Autodesk Inventor part; units mm, degrees
ref_plane "YZ Plane" through (0, 0, 0) normal (1, 0, 0) x (0, 1, 0)
ref_plane "XZ Plane" through (0, 0, 0) normal (0, 1, 0) x (-1, 0, 0)
ref_plane "XY Plane" through (0, 0, 0) normal (0, 0, 1) x (1, 0, 0)
sketch "Sketch1" plane through (0, 0, 0) normal (0, 0, 1) x (1, 0, 0)
  line L0 (0, 0) -> (0, 87.5741)
  line L1 (1.1889, 90.0512) -> (17.8611, 103.4187)
  line L2 (19.05, 105.8958) -> (19.05, 127)
  line L3 (19.05, 127) -> (38.1, 127)
  line L4 (38.1, 127) -> (38.1, 0)
  line L5 (38.1, 0) -> (0, 0)
  arc A0 (17.8611, 103.4187) -> (19.05, 105.8958) centre (15.875, 105.8958) ccw
  arc A1 (1.1889, 90.0512) -> (0, 87.5741) centre (3.175, 87.5741) ccw
  dimension "d0" = 127
  dimension "d1" = 38.1
  dimension "d2" = 19.05
  dimension "d3" = 3.175
revolve "Revolution1" add sketch "Sketch1" angle 360 about axis through (38.1, 127, 0) along (0, -1, 0)
shell "Shell1" thickness 2.54 removed faces 1 at (38.9963, 127, 5.2259)
properties part number "bottle"
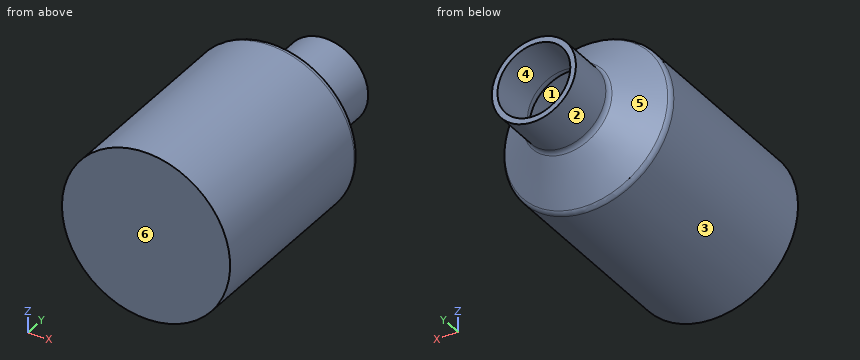
For this review, take the finished solid that the model builds, in its own axes (mm). Face numbers are marked on the shaded views. A direction names the side the tool comes from. Coordinates: 2 decimals unless noted, no trailing zeros. Write each loop counter-clockwise with the first axis right and the second up, starting at its lowest first coordinate (ties: lowest second). Pieces come first, ordered by that corner, then holes. Notation, with made-up numbers: (56, 26.25) - (60, 26.25) arc R5 ccw to (60, 31.25) - close; hole circle Ø1 at (9.5, 6). An arc over 180 degrees is marked (long way). Answer in a Markdown table with one row per item. Add a question column.
Q1. We need section A-A, the plane z = 0. State the section outline as (x, y) points (3 decimals).
Q2. We need section B-B, the plane x = 38.1. State the section outline as (y, z) points (3 decimals), and give its area (3 significant figures).
Q3. For P1, Ø1.5, axis at y = 55.5, z = -29.5, coming from the +X side; P2, Ø8, axis at x = 27.5, y = 52, coming from the -Z side; P3, Ø12, axis at x = 35, y = 86, coming from the +Z side, all flat-tipped, find the tip position at first contact; note any pin that passes through.
Q4. We need section C-C, the plane y = 21. State the section outline as (x, z) points, and give its area (3 significant figures).
Q5. Draft analysis for pull direction Z (two halves, no side actions). For the marked faces 4, 5 and 6, state which applies: +Z half, -Z half, draft (parallel to the pull), parting line (faces both ways), or undercut.
Q6. Tool access review of the marked faces 1, 2 and 3: name each direction out of +Z, -Z, +X, -X, +Y, -Y from which nothing blocks a thin tool from reaching the whole face with its end or side.
Q7. For probe 1 along X at (y, z) = (28, 0); probe 2 along X at (y, z) = (114, 0); probe 3 along Z at (x, y) = (38.1, 52.5), list the stretches that pass through material, from the lowest coordinate up.
Answer list:
| question | item | result |
|---|---|---|
| 1 | outline | (0, 0) - (76.2, 0) - (76.2, 87.574) arc R3.175 ccw to (75.011, 90.051) - (58.339, 103.419) arc R3.175 cw to (57.15, 105.896) - (57.15, 127) - (54.61, 127) - (54.61, 105.896) arc R5.715 ccw to (56.75, 101.437) - (73.422, 88.07) arc R0.635 cw to (73.66, 87.574) - (73.66, 2.54) - (2.54, 2.54) - (2.54, 87.574) arc R0.635 cw to (2.778, 88.07) - (19.45, 101.437) arc R5.715 ccw to (21.59, 105.896) - (21.59, 127) - (19.05, 127) - (19.05, 105.896) arc R3.175 cw to (17.861, 103.419) - (1.189, 90.051) arc R3.175 ccw to (0, 87.574) - close |
| 2 | outline | (0, -38.1) - (87.574, -38.1) arc R3.175 ccw to (90.051, -36.911) - (103.419, -20.239) arc R3.175 cw to (105.896, -19.05) - (127, -19.05) - (127, -16.51) - (105.896, -16.51) arc R5.715 ccw to (101.437, -18.65) - (88.07, -35.322) arc R0.635 cw to (87.574, -35.56) - (2.54, -35.56) - (2.54, 35.56) - (87.574, 35.56) arc R0.635 cw to (88.07, 35.322) - (101.437, 18.65) arc R5.715 ccw to (105.896, 16.51) - (127, 16.51) - (127, 19.05) - (105.896, 19.05) arc R3.175 cw to (103.419, 20.239) - (90.051, 36.911) arc R3.175 ccw to (87.574, 38.1) - (0, 38.1) - close |
| 2 | area | 870 mm2 |
| 3 | P1 | stops at x = 63.1 |
| 3 | P2 | stops at z = -37.52 |
| 3 | P3 | stops at z = 38.1 |
| 4 | outline | circle Ø76.2 at (38.1, 0); hole circle Ø71.12 at (38.1, 0) |
| 4 | area | 588 mm2 |
| 5 | face 4 | undercut |
| 5 | face 5 | parting line |
| 5 | face 6 | draft |
| 6 | face 1 | none |
| 6 | face 2 | +Y |
| 6 | face 3 | +Y, -Y |
| 7 | probe 1 | x = 0 to 2.54, 73.66 to 76.2 |
| 7 | probe 2 | x = 19.05 to 21.59, 54.61 to 57.15 |
| 7 | probe 3 | z = -38.1 to -35.56, 35.56 to 38.1 |
